from build123d import *

# Parameters (mm, degrees)
SKETCH1_R           = 2.1
SKETCH1_W           = 40
SKETCH1_H           = 20
BOSS_EXTRUDE1_DEPTH = 3


with BuildPart() as part:
    # Sketch1 → Boss-Extrude1 (new body)
    with BuildSketch(Plane(origin=(0, 0, 0), x_dir=(1, 0, 0), z_dir=(0, 1, 0))):
        Polygon((0, 0), (-76, 0), (-76, 4), (-79, 4), (-79, 9.5), (-76, 9.5), (-76, 13.5), (-72.9, 13.5), (-72.9, 12.2), (-70.4, 12.2), (-70.4, 13.5), (-66.6, 13.5), (-66.6, 16.5), (-70.4, 16.5), (-70.4, 17.8), (-72.9, 17.8), (-72.9, 16.5), (-76, 16.5), (-76, 20.5), (-79, 20.5), (-79, 26), (-76, 26), (-76, 30), (0, 30), (0, 26), (3, 26), (3, 20.5), (0, 20.5), (0, 16.5), (-3.1, 16.5), (-3.1, 17.8), (-5.6, 17.8), (-5.6, 16.5), (-9.4, 16.5), (-9.4, 13.5), (-5.6, 13.5), (-5.6, 12.2), (-3.1, 12.2), (-3.1, 13.5), (0, 13.5), (0, 9.5), (3, 9.5), (3, 4), (0, 4), align=None)
        with Locations(Location((-19.4, 20.6, 0), (0, 0, 270))):
            Circle(SKETCH1_R, mode=Mode.SUBTRACT)
        with Locations(Location((-68.2, 20.6, 0), (0, 0, 270))):
            Circle(SKETCH1_R, mode=Mode.SUBTRACT)
        with Locations(Location((-68.2, 9.4, 0), (0, 0, 90))):
            Circle(SKETCH1_R, mode=Mode.SUBTRACT)
        with Locations(Location((-19.4, 9.4, 0), (0, 0, 90))):
            Circle(SKETCH1_R, mode=Mode.SUBTRACT)
        with Locations((-43.3, 15)):
            Rectangle(SKETCH1_W, SKETCH1_H, mode=Mode.SUBTRACT)
    extrude(amount=BOSS_EXTRUDE1_DEPTH)


solid = part.part
Check sheet for the modelled part. Datum: model origin and axes. Units: mm. A direction names the side the tool comes from. Coordinates: 2 decimals unless noted, no trailing zeros. Loops run counter-clockwise (first coordinate to the right, second up) from the corner with the lowest first, then second, coordinate; pieces in that order, holes last. Notation, with made-up numbers: (2.5, 37) -> (17.5, 37) arc R18 ccw to (17.5, 69) -> close; hole circle Ø4 at (41, 6). An arc over 180 degrees is marked (long way). Answer in a Markdown table with one row per item.
1. Access from +Z, -Z, +X, -X, +Y, -Y to the whole of each face (thin tool, end or side, straight path). Record for faces 5 (the face through (-77, 1, -20.5)), 6 (the face through (-9.4, 1, -15)), 7 (the face through (0, 1, -2)), 8 (the face through (-78, 1, -26)).
Check values:
| item | result |
|---|---|
| face 5 | -X, +Y, -Y |
| face 6 | +X, +Y, -Y |
| face 7 | +Z, +X, +Y, -Y |
| face 8 | -Z, -X, +Y, -Y |
2. Sectioned sample at A-A, the plane x = -68.2. Record the boundary of the cut face in (y, z), then the cut area to 3 significant figures.
Check values:
| item | result |
|---|---|
| outline | (0, -30) -> (3, -30) -> (3, -22.7) -> (0, -22.7) -> close; (0, -18.5) -> (3, -18.5) -> (3, -16.5) -> (0, -16.5) -> close; (0, -13.5) -> (3, -13.5) -> (3, -11.5) -> (0, -11.5) -> close; (0, -7.3) -> (3, -7.3) -> (3, 0) -> (0, 0) -> close |
| area | 55.8 mm2 |
3. Sectioned sample at B-B, the plane z = -14.5. Record the boundary of the cut face in (x, y).
Check values:
| item | result |
|---|---|
| outline | (-66.6, 0) -> (-63.3, 0) -> (-63.3, 3) -> (-66.6, 3) -> close; (-23.3, 0) -> (-9.4, 0) -> (-9.4, 3) -> (-23.3, 3) -> close |
4. Sectioned sample at D-D, the plane x = -19.4. Record the boundary of the cut face in (y, z).
Check values:
| item | result |
|---|---|
| outline | (0, -30) -> (3, -30) -> (3, -22.7) -> (0, -22.7) -> close; (0, -18.5) -> (3, -18.5) -> (3, -11.5) -> (0, -11.5) -> close; (0, -7.3) -> (3, -7.3) -> (3, 0) -> (0, 0) -> close |
5. Sectioned sample at C-C, the plane x = -54.5. Record the boundary of the cut face in (y, z), then the cut area to 3 significant figures.
Check values:
| item | result |
|---|---|
| outline | (0, -30) -> (3, -30) -> (3, -25) -> (0, -25) -> close; (0, -5) -> (3, -5) -> (3, 0) -> (0, 0) -> close |
| area | 30.0 mm2 |
6. Material ranges on line 1 along X through (y, z) = (2.35, -9.4); line 2 along Z through (x, y) = (-32, 2); line 3 along Z through (x, y) = (-5, 1.6), recorded low to high. Write a range as [from, to].
Check values:
| item | result |
|---|---|
| line 1 | x = [-79, -70.3], [-66.1, -63.3], [-23.3, -21.5], [-17.3, 3] |
| line 2 | z = [-30, -25], [-5, 0] |
| line 3 | z = [-30, -17.8], [-12.2, 0] |
7. Go/stop test with flat-tipped pins: pin 1 (3.5 mm diameter, centred on x = -19.4, z = -9.4, fed in from -Y); pin 2 (0.9 mm diameter, centred on y = 1, z = -28.5, fed in from +X); pin 3 (1.5 mm diameter, centred on x = 1.5, y = 1, fed in from -Z). Record where each tip stops, or that it passes through.
Check values:
| item | result |
|---|---|
| pin 1 | passes through |
| pin 2 | stops at x = 0 |
| pin 3 | stops at z = -26 |
8. Release check for a two-part mould opening along Z. For faces 1 (the face through (-76, 1, -28)), 2 (the face through (1, 1, -26)), 3 (the face through (-74, 1, -16.5)), 4 (the face through (-63.3, 1, -15)) record: released by +Z, released by -Z, zero draft, split by the parting line, or undercut.
Check values:
| item | result |
|---|---|
| face 1 | zero draft |
| face 2 | released by -Z |
| face 3 | undercut |
| face 4 | undercut |
